Can you work these out from the model? Positions are in its coordinate system, mm. Coordinates: 2 decimals unless noted, no trailing zeros. Loops run counter-clockwise (first coordinate to the right, second up) from the corner with the lowest first, then second, coordinate; pieces in that order, holes last.
```python
from build123d import *

# Parameters (mm, degrees)
SKETCH_1_R                   = 19
SKETCH_1_R_2                 = 9.5
EXTRUDE_1_DEPTH              = 5
HOLE_WIZARD_M3_1_D           = 3.2
HOLE_WIZARD_M3_1_CSINK_D     = 6.3
HOLE_WIZARD_M3_1_CSINK_ANGLE = 90


with BuildPart() as part:
    # ｽｹｯﾁ1 → ﾎﾞｽ - 押し出し1 (new body)
    with BuildSketch(Plane.XY):
        Circle(SKETCH_1_R)
        Circle(SKETCH_1_R_2, mode=Mode.SUBTRACT)
    extrude(amount=EXTRUDE_1_DEPTH)

    # M3 丸皿ねじ用皿穴1 (through all)
    with Locations(Plane(origin=(0, 15, 5), x_dir=(1, 0, 0), z_dir=(0, 0, 1))):
        with Locations((0, 0), (15, -15), (0, -30), (-15, -15)):
            CounterSinkHole(HOLE_WIZARD_M3_1_D / 2, HOLE_WIZARD_M3_1_CSINK_D / 2, counter_sink_angle=HOLE_WIZARD_M3_1_CSINK_ANGLE)


solid = part.part
```
Item 1: We'd pull the mould along X, two halves only. Please class faces 1 (the face through (8.767, -16.856, 2.465)), 2 (the face through (0.208, 16.586, 1.701)), 3 (the face through (-9, -4, 0)), 4 (the face through (0.208, -13.414, 1.701)): +X half, -X half, draft (parallel to the pull), parting line (faces both ways), or undercut.
Results are:
face 1: parting line
face 2: undercut
face 3: draft
face 4: undercut
Item 2: Suppose I cut it at A-A, the plane x = 0. Please give me the cut outline in (y, z), plus the area to 3 significant figures.
Results are:
outline: (-19, 0) - (-16.6, 0) - (-16.6, 3.45) - (-18.15, 5) - (-19, 5) - close; (-13.4, 0) - (-9.5, 0) - (-9.5, 5) - (-11.85, 5) - (-13.4, 3.45) - close; (9.5, 0) - (13.4, 0) - (13.4, 3.45) - (11.85, 5) - (9.5, 5) - close; (16.6, 0) - (19, 0) - (19, 5) - (18.15, 5) - (16.6, 3.45) - close
area: 58.2 mm2
Item 3: I'm going to push flat-ended pins straight in: P1, Ø1, axis at x = -1.5, z = 1.5, coming from the -Y side; P2, Ø5, axis at x = -15, y = 0, coming from the +Z side; P3, Ø3.5, axis at x = 0, y = -15, coming from the +Z side. Where does each tip first touch, or does it pass through?
Results are:
P1: stops at y = -18.97
P2: stops at z = 4.35
P3: stops at z = 3.6
Item 4: Suppose I cut it at D-D, the plane y = 8. Please give me the cut outline in (x, z), plus the area to 3 significant figures.
Results are:
outline: (-17.23, 0) - (-5.12, 0) - (-5.12, 5) - (-17.23, 5) - close; (5.12, 0) - (17.23, 0) - (17.23, 5) - (5.12, 5) - close
area: 121 mm2
Item 5: Suppose I cut it at C-C, the plane z = 1.7. Please give me the cut outline in (x, y), plus the area to 3 significant figures.
Results are:
outline: circle Ø38 at (0, 0); hole circle Ø3.2 at (-15, 0); hole circle Ø19 at (0, 0); hole circle Ø3.2 at (0, -15); hole circle Ø3.2 at (0, 15); hole circle Ø3.2 at (15, 0)
area: 818 mm2
Item 6: I need wall thicknesses on line 1 along Y through (x, z) = (0, 1.2); line 2 along X through (y, z) = (-1, 3.9); line 3 along Y through (x, z) = (0, 3.9). Which ranges of each line are inside material? Lowest first, please.
Results are:
line 1: y = -19 to -16.6, -13.4 to -9.5, 9.5 to 13.4, 16.6 to 19
line 2: x = -18.97 to -16.79, -13.21 to -9.45, 9.45 to 13.21, 16.79 to 18.97
line 3: y = -19 to -17.05, -12.95 to -9.5, 9.5 to 12.95, 17.05 to 19
